Geometry check sheet. Reference: the model listing, model coordinates, mm. Round coordinates to 2 decimals unless told otherwise and drop trailing zeros. Write each loop counter-clockwise with the first axis right and the second up, starting at its lowest first coordinate (ties: lowest second). Pieces come first, ordered by that corner, then holes. Notation, with made-up numbers: (-10, 75.25) - (-5, 75.25) arc R11 ccw to (-5, 85.25) - close; hole circle Ø7 at (70, 42). An arc over 180 degrees is marked (long way). Return JSON: item names as keys, results as strings. Group by question number.
from build123d import *

# Parameters (mm, degrees)
F0_R     = 15.85
F0_W     = 18.6
F0_H     = 9.5
F1_DEPTH = 1.5


with BuildPart() as f1:
    # F0 (on Top) → F1 (new body, symmetric)
    with BuildSketch(Plane.XY):
        with BuildLine():
            ThreePointArc((-29.989275, 2.353414), (-33.606886, 0.691253), (-34.863653, -3.086369))
            ThreePointArc((-34.863653, -3.086369), (-30.310889, -17.5), (-20.104701, -28.649625))
            ThreePointArc((-20.104701, -28.649625), (-16.2048, -29.450044), (-12.956521, -27.148181))
            ThreePointArc((-12.956521, -27.148181), (0, -19.85), (12.956521, -27.148181))
            ThreePointArc((12.956521, -27.148181), (16.2048, -29.450044), (20.104701, -28.649625))
            ThreePointArc((20.104701, -28.649625), (30.310889, -17.5), (34.863653, -3.086369))
            ThreePointArc((34.863653, -3.086369), (33.606886, 0.691253), (29.989275, 2.353414))
            ThreePointArc((29.989275, 2.353414), (17.190604, 9.925), (17.032754, 24.794767))
            ThreePointArc((17.032754, 24.794767), (17.402086, 28.758791), (14.758953, 31.735994))
            ThreePointArc((14.758953, 31.735994), (0, 35), (-14.758953, 31.735994))
            ThreePointArc((-14.758953, 31.735994), (-17.402086, 28.758791), (-17.032754, 24.794767))
            ThreePointArc((-17.032754, 24.794767), (-17.190604, 9.925), (-29.989275, 2.353414))
        make_face()
        Polygon((-20.767846, -22.729036), (-30.067846, -6.620964), (-21.840604, -1.870964), (-12.540604, -17.979036), align=None, mode=Mode.SUBTRACT)
        Circle(F0_R, mode=Mode.SUBTRACT)
        Polygon((30.067846, -6.620964), (20.767846, -22.729036), (12.540604, -17.979036), (21.840604, -1.870964), align=None, mode=Mode.SUBTRACT)
        with Locations((0, 24.6)):
            Rectangle(F0_W, F0_H, mode=Mode.SUBTRACT)
    extrude(amount=F1_DEPTH, both=True)


solid = f1.part
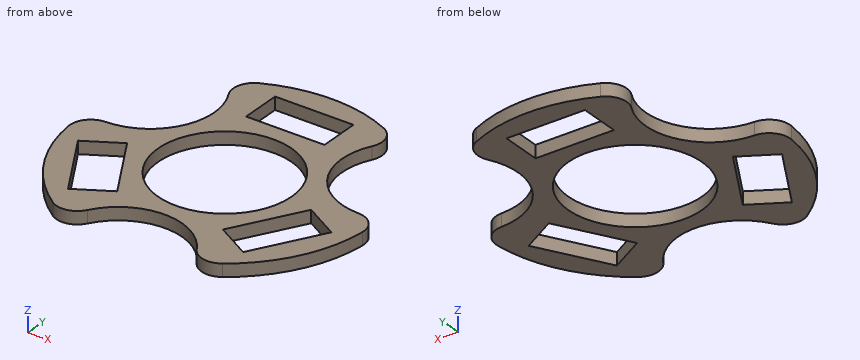
1. Section check D-D (x = 19). Enter the section's corners in (y, z).
2. Section check A-A (x = 0). Enter the section's corners in (y, z), and give its area (4 significant figures).
3. Material ranges on line 1 along Y through (x, z) = (0, -0.1); line 2 along X through (y, z) = (-10, -0.3); line 3 along X through (y, z) = (-19.5, -0.35) (3 decimals), recorded low to high.
4. Section check B-B (z = 0.8). Enter the section's corners in (x, y), and give its area (3 significant figures).
5. Section check C-C (y = 0). Enter the section's corners in (x, z).
6. Depth check by flat-ended pin: pin 1 Ø1.5 at (y, z) = (25, -0.5) entering from +X (3 decimals); pin 2 Ø1.5 at (x, z) = (20.5, 0) entering from -Y; pin 3 Ø0.9 at (x, z) = (2, 0) entering from -Y; pin 4 Ø3 at (x, y) = (-24.5, -6.5) entering from +Z. Enter the tip coordinate at first touch or a pass-through.
Result sheet:
{
 "1": {"outline": "(-29.23, -1.5) - (-21.71, -1.5) - (-21.71, 1.5) - (-29.23, 1.5) - close; (-6.79, -1.5) - (7.42, -1.5) - (7.42, 1.5) - (-6.79, 1.5) - close"},
 "2": {"outline": "(-19.85, -1.5) - (-15.85, -1.5) - (-15.85, 1.5) - (-19.85, 1.5) - close; (15.85, -1.5) - (19.85, -1.5) - (19.85, 1.5) - (15.85, 1.5) - close; (29.35, -1.5) - (35, -1.5) - (35, 1.5) - (29.35, 1.5) - close", "area": "40.95 mm²"},
 "3": {"line 1": "y = -19.85 to -15.85, 15.85 to 19.85, 29.35 to 35", "line 2": "x = -33.54 to -28.12, -17.15 to -12.3, 12.3 to 17.15, 28.12 to 33.54", "line 3": "x = -29.065 to -22.632, -15.175 to 15.175, 22.632 to 29.065"},
 "4": {"outline": "(-34.86, -3.09) arc R35 ccw to (-20.1, -28.65) arc R5 ccw to (-12.96, -27.15) arc R15.15 cw to (12.96, -27.15) arc R5 ccw to (20.1, -28.65) arc R35 ccw to (34.86, -3.09) arc R5 ccw to (29.99, 2.35) arc R15.15 cw to (17.03, 24.79) arc R5 ccw to (14.76, 31.74) arc R35 ccw to (-14.76, 31.74) arc R5 ccw to (-17.03, 24.79) arc R15.15 cw to (-29.99, 2.35) arc R5 ccw to start; hole (-30.07, -6.62) - (-20.77, -22.73) - (-12.54, -17.98) - (-21.84, -1.87) - close; hole circle Ø31.7 at (0, 0); hole (-9.3, 19.85) - (9.3, 19.85) - (9.3, 29.35) - (-9.3, 29.35) - close; hole (12.54, -17.98) - (20.77, -22.73) - (30.07, -6.62) - (21.84, -1.87) - close", "area": "1,510 mm²"},
 "5": {"outline": "(-34.13, -1.5) - (-15.85, -1.5) - (-15.85, 1.5) - (-34.13, 1.5) - close; (15.85, -1.5) - (34.13, -1.5) - (34.13, 1.5) - (15.85, 1.5) - close"},
 "6": {"pin 1": "stops at x = 17.435", "pin 2": "stops at y = -28.88", "pin 3": "stops at y = -20.05", "pin 4": "passes through"}
}
